Verification items for the finished model (mm, model axes). Give positions to 0.01 mm unless a question says otherwise; leave off trailing zeros. Order: outer loops, then holes, each group sorted by start corner. A loop starts at its lowest first (then second) coordinate and runs counter-clockwise, first axis right, second up. Notation, with made-up numbers: (68.25, 68.25) -> (127.25, 68.25) arc R5 cw to (127.25, 74.25) -> close; hole circle Ø5 at (62, 55.25). An arc over 180 degrees is marked (long way). Write each question's results on one line, items separated by ' | '. Start each with the question number.
1. Cross-section at B-B, the plane y = 15.5. Enter the section's corners in (x, z), then the cut area to 3 significant figures.
2. Cross-section at C-C, the plane z = -12. Enter the section's corners in (x, y), then the cut area to 3 significant figures.
3. Material ranges on L1, parallel to Z at x = 17.5, y = 11.5; L2, parallel to Z at x = 26.5, y = 9; L3, parallel to X at y = 1.75, z = 14.5, recorded low to high. Write a range as from..to.
4. Cross-section at D-D, the plane x = 31. Enter the section's corners in (y, z).
5. Mould release check, pull along X, two halves, no side actions. Record for faces 1 (the face through (-7, 17, 0)), 2 (the face through (40.836, 8.381, -4.325)), 3 (the face through (24.854, 8.619, 16.8)): +X half, -X half, draft (parallel to the pull), parting line (faces both ways), or undercut.
6. Cross-section at A-A, the plane z = 20. Enter the section's corners in (x, y), then the cut area to 3 significant figures.
7. Depth check by flat-ended pin: pin 1 Ø3 at (x, y) = (-15.5, 3) entering from -Z; pin 2 Ø3.5 at (y, z) = (9.5, 1) entering from +X; pin 3 Ø1 at (x, y) = (8, 8) entering from +Z. Enter the tip coordinate at first touch or a pass-through.
from build123d import *

# Parameters (mm, degrees)
ESQUISSE1_R             = 40
BOSS_EXTRU_1_DEPTH      = 17
ENL_V_MAT_EXTRU_1_DEPTH = 17
ESQUISSE7_W             = 5.4
ESQUISSE7_H             = 3.1
ENL_V_MAT_EXTRU_3_DEPTH = 20


with BuildPart() as part:
    # Esquisse1 → Boss.-Extru.1 (new body)
    with BuildSketch(Plane(origin=(0, 0, 0), x_dir=(1, 0, 0), z_dir=(0, 1, 0))):
        with Locations(Location((1.175962064, -0.881971548, 0), (0, 0, 270))):
            Circle(ESQUISSE1_R)
    extrude(amount=BOSS_EXTRU_1_DEPTH)

    # Esquisse4 → Enlèv. mat.-Extru.1 (cut)
    with BuildSketch(Plane(origin=(0, 17, 0), x_dir=(1, 0, 0), z_dir=(0, 1, 0))):
        with BuildLine():
            Line((-19.464562445, 22.82828966), (-2.391160411, 7.108611108))
            Line((-2.391160411, 7.108611108), (0, 30))
            ThreePointArc((0, 30), (-10.371868448, 28.150032769), (-19.464562445, 22.82828966))
        make_face()
        with BuildLine():
            ThreePointArc((28.531695489, 9.270509831), (23.567188485, 18.563071591), (15.696113054, 25.566228408))
            Line((15.696113054, 25.566228408), (6.021781713, 4.470810329))
            Line((6.021781713, 4.470810329), (28.531695489, 9.270509831))
        make_face()
        with BuildLine():
            ThreePointArc((17.633557569, -24.270509831), (24.937191951, -16.67742359), (29.165293804, -7.02749154))
            Line((29.165293804, -7.02749154), (6.112826182, -4.345498368))
            Line((6.112826182, -4.345498368), (17.633557569, -24.270509831))
        make_face()
        with BuildLine():
            Line((-2.243847365, -7.156476018), (-17.633557569, -24.270509831))
            ThreePointArc((-17.633557569, -24.270509831), (-8.155156276, -28.870286215), (2.329029809, -29.909457035))
            Line((2.329029809, -29.909457035), (-2.243847365, -7.156476018))
        make_face()
        with BuildLine():
            Line((-7.49960012, -0.077447051), (-28.531695489, 9.270509831))
            ThreePointArc((-28.531695489, 9.270509831), (-29.977355713, -1.165394555), (-27.725874221, -11.457569493))
            Line((-27.725874221, -11.457569493), (-7.49960012, -0.077447051))
        make_face()
    extrude(amount=-ENL_V_MAT_EXTRU_1_DEPTH, mode=Mode.SUBTRACT)

    # Esquisse7 → Enlèv. mat.-Extru.3 (cut)
    with BuildSketch(Plane(origin=(0, 0, 0), x_dir=(-1, 0, 0), z_dir=(0, -1, 0))):
        with Locations((-1.176467364, -1.217534794)):
            Rectangle(ESQUISSE7_W, ESQUISSE7_H)
    extrude(amount=-ENL_V_MAT_EXTRU_3_DEPTH, mode=Mode.SUBTRACT)


solid = part.part
Results below:
1) outline: circle Ø80 at (1.18, 0.88); hole (-28.53, -9.27) -> (-7.5, 0.08) -> (-27.73, 11.46) arc R30 ccw to start; hole (-19.46, -22.83) arc R30 ccw to (0, -30) -> (-2.39, -7.11) -> close; hole (-17.63, 24.27) -> (-2.24, 7.16) -> (2.33, 29.91) arc R30 ccw to start; hole (-1.52, -0.33) -> (3.88, -0.33) -> (3.88, 2.77) -> (-1.52, 2.77) -> close; hole (6.02, -4.47) -> (15.7, -25.57) arc R30 ccw to (28.53, -9.27) -> close; hole (6.11, 4.35) -> (29.17, 7.03) arc R30 ccw to (17.63, 24.27) -> close | area: 3,810 mm²
2) outline: (-36.69, 0) -> (-7.7, 0) -> (-7.7, 17) -> (-36.69, 17) -> close; (-1.88, 0) -> (9.47, 0) -> (9.47, 17) -> (-1.88, 17) -> close; (27.5, 0) -> (39.04, 0) -> (39.04, 17) -> (27.5, 17) -> close | area: 882 mm²
3) L1: z = -35.64..-24.37, -6.92..5.67, 24.04..37.4 | L2: z = -30.08..-14.06, -8.84..6.72, 14.06..31.84 | L3: x = -36.43..-8.85, -0.77..11.98, 26.26..38.79
4) outline: (0, -25.77) -> (17, -25.77) -> (17, 27.54) -> (0, 27.54) -> close
5) face 1: draft | face 2: parting line | face 3: undercut
6) outline: (-33.96, 0) -> (-13.79, 0) -> (-13.79, 17) -> (-33.96, 17) -> close; (0.34, 0) -> (15.16, 0) -> (15.16, 17) -> (0.34, 17) -> close; (22.36, 0) -> (36.31, 0) -> (36.31, 17) -> (22.36, 17) -> close | area: 832 mm²
7) pin 1: stops at z = -36.13 | pin 2: stops at x = 41.18 | pin 3: stops at z = 40.38
